Read the model definition and answer for the solid it produces. Units are mm, in the model's axes. Round coordinates to 2 decimals unless told otherwise and drop trailing zeros. Write each loop counter-clockwise with the first axis right and the second up, starting at its lowest first coordinate (ties: lowest second). Pieces come first, ordered by that corner, then holes.
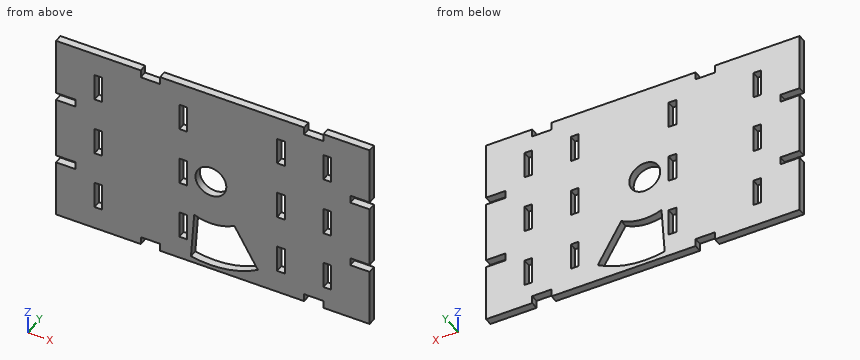
from build123d import *

# Parameters (mm, degrees)
SKETCH2_W           = 100
SKETCH2_H           = 50
SKETCH2_R           = 4
BOSS_EXTRUDE1_DEPTH = 2
SKETCH5_W           = 2
SKETCH5_H           = 7
CUT_EXTRUDE3_DEPTH  = 2
CUT_EXTRUDE6_DEPTH  = 2
SKETCH11_W          = 5
SKETCH11_H          = 2
CUT_EXTRUDE7_DEPTH  = 2
SKETCH12_W          = 9.8
SKETCH12_H          = 50
SKETCH12_W_2        = 8.8
CUT_EXTRUDE8_DEPTH  = 6
SKETCH13_W          = 2
SKETCH13_H          = 7
SKETCH13_W_2        = 5
SKETCH13_H_2        = 2
CUT_EXTRUDE10_DEPTH = 6


with BuildPart() as part:
    # Sketch2 → Boss-Extrude1 (new body)
    with BuildSketch(Plane(origin=(0, 0, 0), x_dir=(1, 0, 0), z_dir=(0, 1, 0))):
        Rectangle(SKETCH2_W, SKETCH2_H)
        with Locations(Location((0, 0, 0), (0, 0, 270))):
            Circle(SKETCH2_R, mode=Mode.SUBTRACT)
    extrude(amount=BOSS_EXTRUDE1_DEPTH)

    # Sketch5 → Cut-Extrude3 (cut)
    with BuildSketch(Plane(origin=(0, 0, 0), x_dir=(-1, 0, 0), z_dir=(0, -1, 0))):
        with Locations((-18.2, -15.5)):
            Rectangle(SKETCH5_W, SKETCH5_H)
        with Locations((-18.2, 0)):
            Rectangle(SKETCH5_W, SKETCH5_H)
        with Locations((-18.2, 15.5)):
            Rectangle(SKETCH5_W, SKETCH5_H)
        with Locations((7.2, 15.5)):
            Rectangle(SKETCH5_W, SKETCH5_H)
        with Locations((7.2, 0)):
            Rectangle(SKETCH5_W, SKETCH5_H)
        with Locations((7.2, -15.5)):
            Rectangle(SKETCH5_W, SKETCH5_H)
    extrude(amount=-CUT_EXTRUDE3_DEPTH, mode=Mode.SUBTRACT)

    # Sketch10 → Cut-Extrude6 (cut)
    with BuildSketch(Plane(origin=(0, 2, 0), x_dir=(1, 0, 0), z_dir=(0, 1, 0))):
        with BuildLine():
            ThreePointArc((-5.171573663, 23.436186248), (3.772267489, 23.701687661), (12.191771414, 20.672704462))
            Line((12.191771414, 20.672704462), (6.095885707, 10.336352231))
            ThreePointArc((6.095885707, 10.336352231), (0.977437683, 11.960126069), (-4.336736478, 11.188955122))
            Line((-4.336736478, 11.188955122), (-5.171573663, 23.436186248))
        make_face()
    extrude(amount=-CUT_EXTRUDE6_DEPTH, mode=Mode.SUBTRACT)

    # Sketch11 → Cut-Extrude7 (cut)
    with BuildSketch(Plane(origin=(0, 2, 0), x_dir=(1, 0, 0), z_dir=(0, 1, 0))):
        with Locations((-15.7, -24)):
            Rectangle(SKETCH11_W, SKETCH11_H)
        with Locations((26.7, -24)):
            Rectangle(SKETCH11_W, SKETCH11_H)
        with Locations((26.7, 24)):
            Rectangle(SKETCH11_W, SKETCH11_H)
        with Locations((-15.7, 24)):
            Rectangle(SKETCH11_W, SKETCH11_H)
    extrude(amount=-CUT_EXTRUDE7_DEPTH, mode=Mode.SUBTRACT)

    # Sketch12 → Cut-Extrude8 (cut)
    with BuildSketch(Plane(origin=(0, 2, 0), x_dir=(1, 0, 0), z_dir=(0, 1, 0))):
        with Locations((-45.1, 0)):
            Rectangle(SKETCH12_W, SKETCH12_H)
        with Locations((45.6, 0)):
            Rectangle(SKETCH12_W_2, SKETCH12_H)
    extrude(amount=-CUT_EXTRUDE8_DEPTH, mode=Mode.SUBTRACT)

    # Sketch13 → Cut-Extrude10 (cut)
    with BuildSketch(Plane(origin=(0, 2, 0), x_dir=(1, 0, 0), z_dir=(0, 1, 0))):
        with Locations((-29.2, 15.5)):
            Rectangle(SKETCH13_W, SKETCH13_H)
        with Locations((-29.2, 0)):
            Rectangle(SKETCH13_W, SKETCH13_H)
        with Locations((-29.2, -15.5)):
            Rectangle(SKETCH13_W, SKETCH13_H)
        with Locations((30.2, 15.5)):
            Rectangle(SKETCH13_W, SKETCH13_H)
        with Locations((30.2, 0)):
            Rectangle(SKETCH13_W, SKETCH13_H)
        with Locations((30.2, -15.5)):
            Rectangle(SKETCH13_W, SKETCH13_H)
        with Locations((-37.7, 9)):
            Rectangle(SKETCH13_W_2, SKETCH13_H_2)
        with Locations((-37.7, -9)):
            Rectangle(SKETCH13_W_2, SKETCH13_H_2)
        with Locations((38.7, 9)):
            Rectangle(SKETCH13_W_2, SKETCH13_H_2)
        with Locations((38.7, -9)):
            Rectangle(SKETCH13_W_2, SKETCH13_H_2)
    extrude(amount=-CUT_EXTRUDE10_DEPTH, mode=Mode.SUBTRACT)


solid = part.part
Q1. Section B-B (x = 0) is taken. Determine the outline of the cut face in (y, z).
Verdict:
outline: (0, -25) - (2, -25) - (2, -24) - (0, -24) - close; (0, -12) - (2, -12) - (2, -4) - (0, -4) - close; (0, 4) - (2, 4) - (2, 25) - (0, 25) - close
Q2. Straight lines are drawn through the part: probe 1 along X at (y, z) = (0.45, 0); probe 2 along X at (y, z) = (1.35, -18); probe 3 along Z at (x, y) = (10.5, 0.9). For each, find the intervals that lie inside material, in ascending order.
Verdict:
probe 1: x = -40.2 to -30.2, -28.2 to -8.2, -6.2 to -4, 4 to 17.2, 19.2 to 29.2, 31.2 to 41.2
probe 2: x = -40.2 to -30.2, -28.2 to -8.2, -6.2 to -4.8, 10.62 to 17.2, 19.2 to 29.2, 31.2 to 41.2
probe 3: z = -25 to -21.58, -17.8 to 25
Q3. Section C-C (y = 1) is taken. State how many separate pieces and enclosed holes the cut face has, then the cut area to 3 significant figures.
Verdict:
separate pieces: 1
enclosed holes: 14
area: 3,600 mm2
Q4. Section A-A (z = 0) is taken. Determine the outline of the cut face in (x, y).
Verdict:
outline: (-40.2, 0) - (-30.2, 0) - (-30.2, 2) - (-40.2, 2) - close; (-28.2, 0) - (-8.2, 0) - (-8.2, 2) - (-28.2, 2) - close; (-6.2, 0) - (-4, 0) - (-4, 2) - (-6.2, 2) - close; (4, 0) - (17.2, 0) - (17.2, 2) - (4, 2) - close; (19.2, 0) - (29.2, 0) - (29.2, 2) - (19.2, 2) - close; (31.2, 0) - (41.2, 0) - (41.2, 2) - (31.2, 2) - close
Q5. Section D-D (z = -14.5) is taken. Determine the outline of the cut face in (x, y), then the cut area to 3 significant figures.
Verdict:
outline: (-40.2, 0) - (-30.2, 0) - (-30.2, 2) - (-40.2, 2) - close; (-28.2, 0) - (-8.2, 0) - (-8.2, 2) - (-28.2, 2) - close; (-6.2, 0) - (-4.56, 0) - (-4.56, 2) - (-6.2, 2) - close; (8.55, 0) - (17.2, 0) - (17.2, 2) - (8.55, 2) - close; (19.2, 0) - (29.2, 0) - (29.2, 2) - (19.2, 2) - close; (31.2, 0) - (41.2, 0) - (41.2, 2) - (31.2, 2) - close
area: 121 mm2
